The listing builds one solid part. Answer for the finished solid, in the listing's coordinates (mm). Give positions to 0.01 mm unless a question says otherwise; leave off trailing zeros. Loops run counter-clockwise (first coordinate to the right, second up) from the corner with the lowest first, then second, coordinate; pieces in that order, holes last. Notation, with made-up numbers: (59.25, 78) - (94.25, 78) arc R7 ccw to (94.25, 89) - close; hole circle Ø5 at (-29, 72). An arc over 180 degrees is marked (long way). One line per item, written item: value. Start each with the question number.
from build123d import *

# Parameters (mm, degrees)
F0_R     = 12.7
F1_DEPTH = 25.4


with BuildPart() as f1:
    # F0 (on Top) → F1 (new body)
    with BuildSketch(Plane.XY):
        with BuildLine():
            ThreePointArc((31.75, 63.5), (0, 31.75), (31.75, 0))
            Line((31.75, 0), (136.525, 0))
            Line((136.525, 0), (136.525, 31.75))
            ThreePointArc((136.525, 31.75), (114.07436, 41.04936), (104.775, 63.5))
            Line((104.775, 63.5), (31.75, 63.5))
        make_face()
        with Locations((31.75, 31.75)):
            Circle(F0_R, mode=Mode.SUBTRACT)
    extrude(amount=F1_DEPTH)


solid = f1.part
1. Flat-ended cylindrical pins translate along their axes: pin 1 (3 mm diameter, centred on y = 32.5, z = 7, fed in from -X); pin 2 (3 mm diameter, centred on x = 112.5, z = 8, fed in from -Y); pin 3 (10 mm diameter, centred on y = 41.5, z = 20.5, fed in from -X). Find the tip coordinate at first contact, or state that the pin passes through.
2. Determine the mould class of faces 1 (the flat face through (67, 32, 25.4)), 2 (the cylindrical face through (0, 32, 13)), 3 (the cylindrical face through (37.61, 20.483, 12.522)), 4 (the cylindrical face through (114.323, 40.804, 12.522)) for opening direction X: released by +X, released by -X, zero draft, split by the parting line, or undercut.
3. A cutting plane is placed at C-C (x = 38). Determine the outline of the cut face in (y, z).
4. A cutting plane is placed at A-A (y = 36.5). Determine the outline of the cut face in (x, z), plus the area to 3 significant figures.
5. A cutting plane is placed at D-D (x = 15). Determine the outline of the cut face in (y, z), plus the area to 3 significant figures.
6. Find the intervals of material crossed by L1, parallel to Y at x = 31.75, z = 6.25; L2, parallel to X at y = 39.5, z = 7.75; L3, parallel to Y at x = 107.5, z = 19.5, in increasing order. Write a range as [from, to].
7. A cutting plane is placed at B-B (z = 11.5). Determine the outline of the cut face in (x, y) (3 decimals).
Results below:
1. pin 1: stops at x = 0
1. pin 2: stops at y = 0
1. pin 3: stops at x = 0.36
2. face 1: zero draft
2. face 2: released by -X
2. face 3: undercut
2. face 4: released by +X
3. outline: (0, 0) - (20.69, 0) - (20.69, 25.4) - (0, 25.4) - close; (42.81, 0) - (63.5, 0) - (63.5, 25.4) - (42.81, 25.4) - close
4. outline: (0.36, 0) - (19.97, 0) - (19.97, 25.4) - (0.36, 25.4) - close; (43.53, 0) - (119.82, 0) - (119.82, 25.4) - (43.53, 25.4) - close
4. area: 2,440 mm^2
5. outline: (4.78, 0) - (58.72, 0) - (58.72, 25.4) - (4.78, 25.4) - close
5. area: 1,370 mm^2
6. L1: y = [0, 19.05], [44.45, 63.5]
6. L2: x = [0.96, 21.69], [41.81, 115.74]
6. L3: y = [0, 50.63]
7. outline: (31.75, 0) - (136.525, 0) - (136.525, 31.75) arc R31.75 cw to (104.775, 63.5) - (31.75, 63.5) arc R31.75 ccw to start; hole circle Ø25.4 at (31.75, 31.75)
